from build123d import *

# Parameters (mm, degrees)
SKETCH_1_R               = 4
EXTRUDE_1_DEPTH          = 1.4
CUT_EXTRUDE_1_DEPTH      = 61.639013844
CUT_EXTRUDE_1_DEPTH_BACK = 61.639013844
SKETCH_2_W               = 23.6
SKETCH_2_H               = 12.6
SKETCH_2_R               = 1.5
CUT_EXTRUDE_2_DEPTH      = 61.639013844
CUT_EXTRUDE_2_DEPTH_BACK = 61.639013844
SKETCH_3_R               = 1.5
SKETCH_3_R_2             = 1.499999999
SKETCH_3_R_3             = 1.500000004


with BuildPart() as part:
    # Эскиз1 → Бобышка-Вытянуть1 (new, symmetric)
    with BuildSketch(Plane.XY):
        Polygon((-55.1, 15), (-49.49, 15), (-49.49, 17.8), (-41.49, 17.8), (-41.49, 15), (-31.16, 15), (-31.16, 17.8), (-23.16, 17.8), (-23.16, 15), (-12.83, 15), (-12.83, 17.8), (-4.83, 17.8), (-4.83, 15), (5.5, 15), (5.5, 17.8), (13.5, 17.8), (13.5, 15), (23.83, 15), (23.83, 17.8), (31.83, 17.8), (31.83, 15), (42.16, 15), (42.16, 17.8), (50.16, 17.8), (50.16, 15), (55.1, 15), (55.1, 11.5), (57.9, 11.5), (57.9, 6.5), (55.1, 6.5), (55.1, 5), (55.1, -5), (55.1, -6.5), (57.9, -6.5), (57.9, -11.5), (55.1, -11.5), (55.1, -15), (50.16, -15), (50.16, -17.8), (42.16, -17.8), (42.16, -15), (31.83, -15), (31.83, -17.8), (23.83, -17.8), (23.83, -15), (13.5, -15), (13.5, -17.8), (5.5, -17.8), (5.5, -15), (-4.83, -15), (-4.83, -17.8), (-12.83, -17.8), (-12.83, -15), (-23.16, -15), (-23.16, -17.8), (-31.16, -17.8), (-31.16, -15), (-41.49, -15), (-41.49, -17.8), (-49.49, -17.8), (-49.49, -15), (-55.1, -15), (-57.9, -15), (-57.9, -12), (-55.1, -12), (-55.1, -11.5), (-55.1, -6.5), (-55.1, -5), (-55.1, 5), (-55.1, 6.5), (-55.1, 11.5), (-55.1, 12), (-57.9, 12), (-57.9, 15), align=None)
        with Locations((5, 0)):
            Circle(SKETCH_1_R, mode=Mode.SUBTRACT)
        with Locations((-49, 0)):
            Circle(SKETCH_1_R, mode=Mode.SUBTRACT)
    extrude(amount=EXTRUDE_1_DEPTH, both=True)

    # Эскиз2 → Вырез-Вытянуть1 (cut, two sides: drawn at the far end of the back side and taken through both)
    with BuildSketch(Plane(origin=(0, 0, -1.4), x_dir=(-1, 0, 0), z_dir=(0, 0, -1)).offset(-CUT_EXTRUDE_1_DEPTH_BACK)):
        with Locations((22, 0)):
            Rectangle(SKETCH_2_W, SKETCH_2_H)
        with Locations((8.565, 0)):
            Circle(SKETCH_2_R)
        with Locations((35.435, 0)):
            Circle(SKETCH_2_R)
    extrude(amount=CUT_EXTRUDE_1_DEPTH + CUT_EXTRUDE_1_DEPTH_BACK, mode=Mode.SUBTRACT)

    # Эскиз3 → Вырез-Вытянуть2 (cut, two sides: drawn at the far end of the back side and taken through both)
    with BuildSketch(Plane(origin=(0, 0, -1.4), x_dir=(-1, 0, 0), z_dir=(0, 0, -1)).offset(-CUT_EXTRUDE_2_DEPTH_BACK)):
        with Locations((31.667851618, -11.228512478)):
            Circle(SKETCH_3_R)
        with Locations((-48.429379636, -8.299999991)):
            Circle(SKETCH_3_R_2)
        with Locations((-15.648202479, -11.743667469)):
            Circle(SKETCH_3_R_2)
        with Locations((39.99236744, 10.8145639)):
            Circle(SKETCH_3_R)
        with Locations((-36.253127984, 10.284376689)):
            Circle(SKETCH_3_R_3)
    extrude(amount=CUT_EXTRUDE_2_DEPTH + CUT_EXTRUDE_2_DEPTH_BACK, mode=Mode.SUBTRACT)


solid = part.part
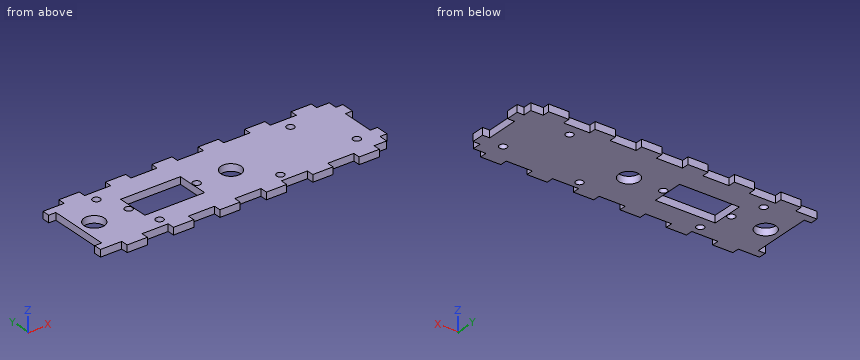
Here's how the part is built. I have some questions about the finished solid (model axes, mm). Round coordinates to 2 decimals unless told otherwise and drop trailing zeros. Order: outer loops, then holes, each group sorted by start corner. A loop starts at its lowest first (then second) coordinate and runs counter-clockwise, first axis right, second up. Notation, with made-up numbers: M -36,31 L 13,31 A29 ccw 13,67 Z; hole C 57.25,-36 d3. An arc over 180 degrees is marked long. One line per question, with ' | ' between items.
1) Imagine slicing it at D-D, the plane z = 0.55. Count the separate pieces of the cut face and the enclosed holes in it, plus the area to 3 significant figures.
Checked values:
separate pieces: 1 | enclosed holes: 10 | area: 3,170 mm²
2) Imagine slicing it at B-B, the plane y = -8.3. Write out the boundary of the cut face in (x, z), plus the area to 3 significant figures.
Checked values:
outline: M -55.1,-1.4 L 46.93,-1.4 L 46.93,1.4 L -55.1,1.4 Z; M 49.93,-1.4 L 57.9,-1.4 L 57.9,1.4 L 49.93,1.4 Z | area: 308 mm²
3) Imagine slicing it at C-C, the plane x = -3. Write out the boundary of the cut face in (y, z).
Checked values:
outline: M -15,-1.4 L 15,-1.4 L 15,1.4 L -15,1.4 Z
4) I need wall thicknesses on line 1 (X direction, y = -16, z = 0.45); line 2 (X direction, y = 3.5, z = -1.15); line 3 (Y direction, x = -49, z = -0.25). Which ranges of each line are inside material? Lowest first, please.
Checked values:
line 1: x = -49.49 to -41.49, -31.16 to -23.16, -12.83 to -4.83, 5.5 to 13.5, 23.83 to 31.83, 42.16 to 50.16 | line 2: x = -55.1 to -50.94, -47.06 to -33.8, -10.2 to 3.06, 6.94 to 55.1 | line 3: y = -17.8 to -4, 4 to 17.8
5) I'm going to push flat-ended pins straight in: pin 1 Ø1.4 at (y, z) = (5, 0.5) entering from -X; pin 2 Ø0.8 at (y, z) = (-16.5, 0.5) entering from +X; pin 3 Ø1.4 at (y, z) = (-17, -0.5) entering from -X. Where does each tip first touch, or does it pass through?
Checked values:
pin 1: stops at x = -55.1 | pin 2: stops at x = 50.16 | pin 3: stops at x = -49.49
6) Imagine slicing it at A-A, the plane y = 0. Write out the boundary of the cut face in (x, z) (3 decimals), plus the area to 3 significant figures.
Checked values:
outline: M -55.1,-1.4 L -53,-1.4 L -53,1.4 L -55.1,1.4 Z; M -45,-1.4 L -36.935,-1.4 L -36.935,1.4 L -45,1.4 Z; M -33.935,-1.4 L -33.8,-1.4 L -33.8,1.4 L -33.935,1.4 Z; M -10.2,-1.4 L -10.065,-1.4 L -10.065,1.4 L -10.2,1.4 Z; M -7.065,-1.4 L 1,-1.4 L 1,1.4 L -7.065,1.4 Z; M 9,-1.4 L 55.1,-1.4 L 55.1,1.4 L 9,1.4 Z | area: 181 mm²
